```python
from build123d import *

# Parameters (mm, degrees)
EXTRUDE_1_DEPTH     = 45
SKETCH_2_R          = 2.5
EXTRUDE_2_DEPTH     = 7
CHAMFER_1_SIZE      = 0.5
SKETCH_3_R          = 2.5
CUT_EXTRUDE_1_DEPTH = 7


with BuildPart() as part:
    # 草图1 → 凸台-拉伸1 (new body)
    with BuildSketch(Plane(origin=(0, 0, 0), x_dir=(0, 0, -1), z_dir=(1, 0, 0))):
        Polygon((2.747304238, -2.88484305), (3.871999486, 0.936813737), (1.124695248, 3.821656787), (-2.747304238, 2.88484305), (-3.871999486, -0.936813737), (-1.124695248, -3.821656787), align=None)
    extrude(amount=EXTRUDE_1_DEPTH)

    # 草图2 → 凸台-拉伸2 (add)
    with BuildSketch(Plane(origin=(45, 0, 0), x_dir=(0, 0, -1), z_dir=(1, 0, 0))):
        Circle(SKETCH_2_R)
    extrude(amount=EXTRUDE_2_DEPTH)

    # 倒角1
    chamfer_1_edges = [part.edges().sort_by_distance(p)[0] for p in [
        (52, 0, 2.5),
    ]]
    chamfer(chamfer_1_edges, length=CHAMFER_1_SIZE)

    # 草图3 → 切除-拉伸1 (cut)
    with BuildSketch(Plane.ZY):
        with Locations(Location((0, 0, 0), (0, 0, 180))):
            Circle(SKETCH_3_R)
    extrude(amount=-CUT_EXTRUDE_1_DEPTH, mode=Mode.SUBTRACT)


solid = part.part
```
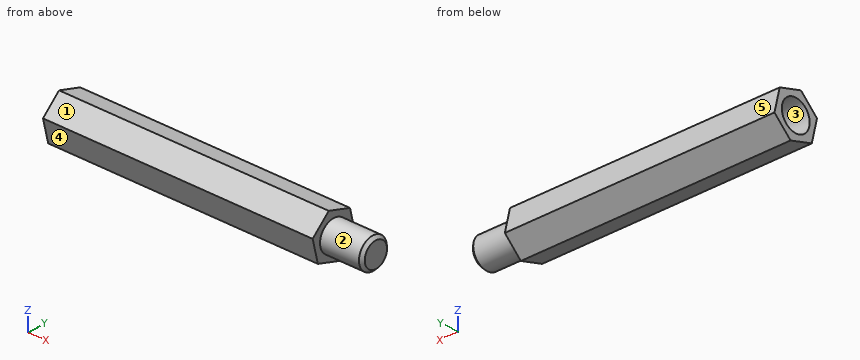
The listing builds one solid part. Answer for the finished solid, in the listing's coordinates (mm). Face numbers are marked on the shaded views. A direction names the side the tool comes from. Coordinates: 2 decimals unless noted, no trailing zeros. Write each loop counter-clockwise with the first axis right and the second up, starting at its lowest first coordinate (ties: lowest second). Pieces come first, ordered by that corner, then holes. Notation, with made-up numbers: (61, 34) - (113, 34) arc R13 ccw to (113, 58) - close; hole circle Ø2 at (-30, 83). An arc over 180 degrees is marked (long way). One line per item, written item: value.
1) Find section D-D (z = 0). Give the vertices of the cut face in (x, y), and give its area (3 significant figures).
Geometry check:
outline: (0, -3.55) - (45, -3.55) - (45, -2.5) - (51.5, -2.5) - (52, -2) - (52, 2) - (51.5, 2.5) - (45, 2.5) - (45, 3.55) - (0, 3.55) - (0, 2.5) - (7, 2.5) - (7, -2.5) - (0, -2.5) - close
area: 319 mm2
2) Consider line 1 along X through (y, z) = (1.5, 2.5); line 2 along X through (y, z) = (1.5, -0.25); line 3 along Y through (x, z) = (5.5, -0.5). Determine where each line is inside the solid, lowest interval first. Write a range as from..to.
Geometry check:
line 1: x = 0..45
line 2: x = 7..52
line 3: y = -3.43..-2.45, 2.45..3.67
3) Find section A-A (x = 4). Give the vertices of the cut face in (y, z), and give its area (3 significant figures).
Geometry check:
outline: (-3.82, 1.12) - (-2.88, -2.75) - (0.94, -3.87) - (3.82, -1.12) - (2.88, 2.75) - (-0.94, 3.87) - close; hole circle Ø5 at (0, 0)
area: 21.6 mm2
4) For a pull along Z with two mould halves and no side action, classify the marked faces 3, 4 and 5 as pulls with the +Z half, pulls with the -Z half, needs draft (parallel to the pull), parting line crosses it, or undercut.
Geometry check:
face 3: undercut
face 4: pulls with the -Z half
face 5: pulls with the +Z half
5) A tool of negligible diameter and unlimited length cuts with its end or side. For the marked faces 1 and 2, from which of +Z, -Z, +X, -X, +Y, -Y can it reach the whole face along a straight path? Write none if from no direction.
Geometry check:
face 1: +Z, +X, -X, -Y
face 2: +X
6) Find section B-B (x = 19.5). Give the vertices of the cut face in (y, z), and give its area (3 significant figures).
Geometry check:
outline: (-3.82, 1.12) - (-2.88, -2.75) - (0.94, -3.87) - (3.82, -1.12) - (2.88, 2.75) - (-0.94, 3.87) - close
area: 41.2 mm2
7) Find section C-C (y = 0). Give the vertices of the cut face in (x, z).
Geometry check:
outline: (0, -3.6) - (45, -3.6) - (45, -2.5) - (51.5, -2.5) - (52, -2) - (52, 2) - (51.5, 2.5) - (45, 2.5) - (45, 3.6) - (0, 3.6) - (0, 2.5) - (7, 2.5) - (7, -2.5) - (0, -2.5) - close
8) Each of these flat-tipped pins is pushed along its axis until it touches: pin 1 Ø4 at (x, z) = (28, 3) entering from -Y; pin 2 Ø3 at (y, z) = (0, 0) entering from -X. Where does it stop, or does it pass through?
Geometry check:
pin 1: stops at y = -3.82
pin 2: stops at x = 7
